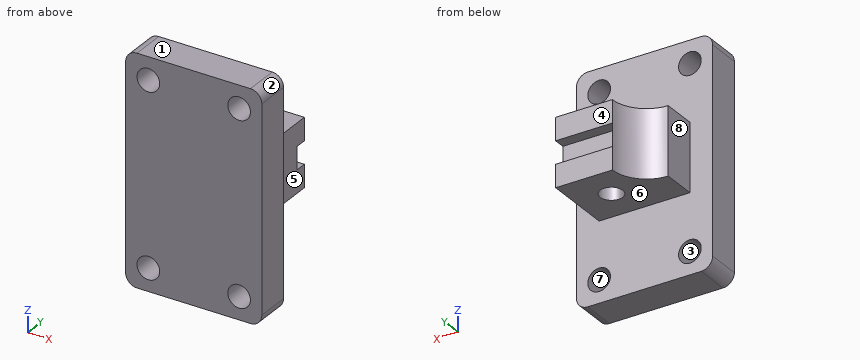
Autodesk Inventor part; units mm, degrees
ref_plane "YZ Plane" through (0, 0, 0) normal (1, 0, 0) x (0, 1, 0)
ref_plane "XZ Plane" through (0, 0, 0) normal (0, 1, 0) x (-1, 0, 0)
ref_plane "XY Plane" through (0, 0, 0) normal (0, 0, 1) x (1, 0, 0)
sketch "Sketch1" plane through (0, 0, 0) normal (0, 0, 1) x (1, 0, 0)
  line L0 (0, 0) -> (50.8, 0)
  line L1 (50.8, 0) -> (50.8, 38.1)
  line L2 (50.8, 38.1) -> (19.05, 38.1)
  line L3 (0, 19.05) -> (0, 0)
  arc A0 (0, 19.05) -> (19.05, 38.1) centre (0, 38.1) ccw
  circle A1 centre (31.75, 19.05) radius 6.35
  dimension "d0" = 38.1
  dimension "d1" = 50.8
  dimension "d4" = 19.05
  dimension "d5" = 12.7
  dimension "d6" = 19.05
  dimension "d7" = 19.05
extrude "Extrusion1" add sketch "Sketch1" along normal blind 38.1
sketch "Sketch2" plane through (0, 0, 0) normal (0, -1, 0) x (1, 0, 0)
  line L0 (57.15, 82.55) -> (-6.35, 82.55)
  line L1 (-12.7, 76.2) -> (-12.7, -38.1)
  line L2 (-6.35, -44.45) -> (57.15, -44.45)
  line L3 (63.5, -38.1) -> (63.5, 76.2)
  line L4 (0, 0) -> (0, 38.1)
  line L5 (0, 0) -> (50.8, 0)
  arc A0 (63.5, 76.2) -> (57.15, 82.55) centre (57.15, 76.2) ccw
  arc A1 (-6.35, 82.55) -> (-12.7, 76.2) centre (-6.35, 76.2) ccw
  arc A2 (-12.7, -38.1) -> (-6.35, -44.45) centre (-6.35, -38.1) ccw
  arc A3 (57.15, -44.45) -> (63.5, -38.1) centre (57.15, -38.1) ccw
  circle A4 centre (50.8, -31.75) radius 6.35
  circle A5 centre (0, -31.75) radius 6.35
  circle A6 centre (50.8, 69.85) radius 6.35
  circle A7 centre (0, 69.85) radius 6.35
  point P0 (-12.7, -44.45)
  point P1 (-12.7, 82.55)
  point P2 (63.5, -44.45)
  dimension "d11" = 76.2
  dimension "d12" = 127
  dimension "d13" = 12.7
  dimension "d14" = 44.45
  dimension "d15" = 6.35
  dimension "d16" = 12.7
  dimension "d17" = 12.7
  dimension "d18" = 12.7
extrude "Extrusion2" add sketch "Sketch2" along normal blind 19.05
sketch "Sketch3" plane through (19.05, 38.1, 0) normal (0, 1, 0) x (1, 0, 0)
  line L0 (31.75, 0) -> (31.75, -38.1)
  line L1 (0, 0) -> (0, -38.1)
  line L2 (31.75, -12.7) -> (0, -12.7)
  line L3 (0, -12.7) -> (0, -25.4)
  line L4 (0, -25.4) -> (31.75, -25.4)
  line L5 (31.75, -25.4) -> (31.75, -12.7)
  point P0 (-19.05, 0)
  dimension "d21" = 12.7
  dimension "d22" = 12.7
extrude "Extrusion3" cut sketch "Sketch3" against normal blind 6.35
properties part number "HW 8 Part6"
CAD build for the part. Positions are in the model's coordinates, mm. Face numbers are marked on the shaded views. A direction names the side the tool comes from. Round coordinates to 2 decimals unless told otherwise and drop trailing zeros. Write each loop counter-clockwise with the first axis right and the second up, starting at its lowest first coordinate (ties: lowest second). Pieces come first, ordered by that corner, then holes.
(1) Slice it at D-D, the plane x = 41.5. Write the cut outline in (y, z).
(2) Slice it at A-A, the plane x = 31.75. Write the cut outline in (y, z).
(3) 3-axis set-ups, long thin cutter, end or side, ignore diameter. For the marked faces 4, 5, 6, 7 and 8: which of +Z, -Z, +X, -X, +Y, -Y reach the whole face in a straight line?
(4) Slice it at C-C, the plane y = -13. Write the cut outline in (x, z), and give its area (3 significant figures).
(5) Probe line 1 along Z through (x, y) = (0, -11); line 2 along Y through (x, z) = (31.5, 7.5); line 3 along X through (y, z) = (-5, 69). List the from-to ranges inside material, lowest first.
(6) Mould opens along X. For the marked faces 1, 2 and 3 say: pulls with the +X half, pulls with the -X half, needs draft (parallel to the pull), parting line crosses it, or undercut.
(7) Slice it at B-B, the plane z = -31.75. Write the cut outline in (x, y).
(8) Drop flat-ended pins along their axis: P1, Ø11.5, axis at x = 35, y = 28, coming from the -Z side; P2, Ø6, axis at x = 54, z = -6.5, coming from the +Y side; P3, Ø10, axis at x = 50.8, z = -31.75, coming from the +Y side; P4, Ø7, axis at x = 41, y = 35.5, coming from the +Z side. Give the stop position or say it passes through.
From the geometry:
1. outline: (-19.05, -44.45) - (0, -44.45) - (0, 0) - (38.1, 0) - (38.1, 12.7) - (31.75, 12.7) - (31.75, 25.4) - (38.1, 25.4) - (38.1, 38.1) - (0, 38.1) - (0, 82.55) - (-19.05, 82.55) - close
2. outline: (-19.05, -44.45) - (0, -44.45) - (0, 0) - (12.7, 0) - (12.7, 38.1) - (0, 38.1) - (0, 82.55) - (-19.05, 82.55) - close; (25.4, 0) - (38.1, 0) - (38.1, 12.7) - (31.75, 12.7) - (31.75, 25.4) - (38.1, 25.4) - (38.1, 38.1) - (25.4, 38.1) - close
3. face 4: +Z, -Z, +X, -X, +Y
3. face 5: +Z, -Z, +X, +Y
3. face 6: -Z, +X, -X, +Y
3. face 7: +Y, -Y
3. face 8: +Z, -Z, -X, +Y
4. outline: (-12.7, -38.1) arc R6.35 ccw to (-6.35, -44.45) - (57.15, -44.45) arc R6.35 ccw to (63.5, -38.1) - (63.5, 76.2) arc R6.35 ccw to (57.15, 82.55) - (-6.35, 82.55) arc R6.35 ccw to (-12.7, 76.2) - close; hole circle Ø12.7 at (0, -31.75); hole circle Ø12.7 at (0, 69.85); hole circle Ø12.7 at (50.8, -31.75); hole circle Ø12.7 at (50.8, 69.85)
4. area: 9,140 mm2
5. line 1: z = -44.45 to -38.1, -25.4 to 63.5, 76.2 to 82.55
5. line 2: y = -19.05 to 12.7, 25.4 to 38.1
5. line 3: x = -12.7 to -6.29, 6.29 to 44.51, 57.09 to 63.5
6. face 1: needs draft
6. face 2: pulls with the +X half
6. face 3: undercut
7. outline: (-12.7, -19.05) - (-6.35, -19.05) - (-6.35, 0) - (-12.7, 0) - close; (6.35, -19.05) - (44.45, -19.05) - (44.45, 0) - (6.35, 0) - close; (57.15, -19.05) - (63.5, -19.05) - (63.5, 0) - (57.15, 0) - close
8. P1: stops at z = 0
8. P2: stops at y = 0
8. P3: passes through
8. P4: stops at z = 38.1
